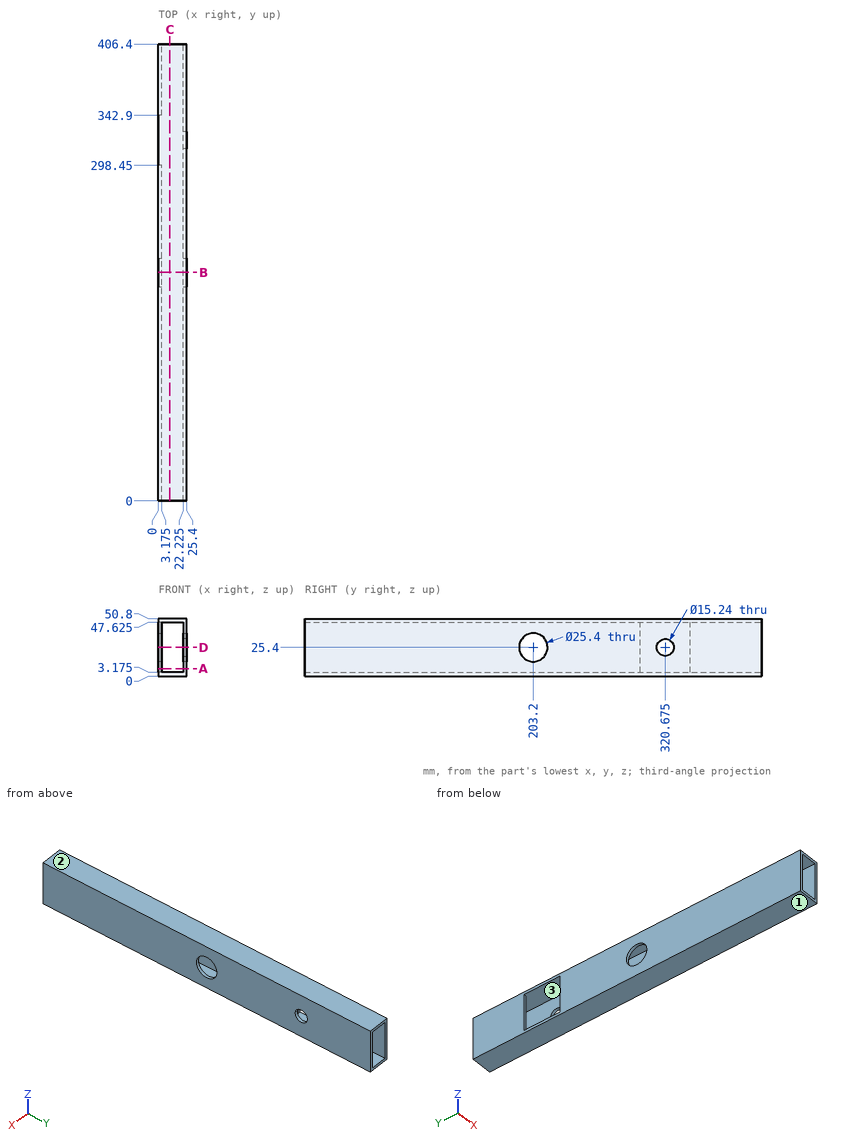
For this review, use the dimensioned drawing (mm, ordinates from the lowest corner) and the shaded views. Coordinates: 2 decimals unless noted, no trailing zeros. Loops run counter-clockwise (first coordinate to the right, second up) from the corner with the lowest first, then second, coordinate; pieces in that order, holes last. Notation, with made-up numbers: (1, -31.5) -> (57, -31.5) arc R21 ccw to (57, 7.5) -> close; hole circle Ø5 at (2, 30). An arc over 180 degrees is marked (long way). Use a Markdown table: item, result. Add a question column.
Item 1: The part is to be moulded in two halves that separate along Z. For the marked faces 1, 2 and 3, say which applies: +Z half, -Z half, draft (parallel to the pull), parting line (faces both ways), or undercut.
Item 2: We need section D-D, the plane z = 25.4. Write out the cut boundary in (x, y) (3 decimals), and give its area (3 significant figures).
Item 3: We need section C-C, the plane x = 10.25. Write out the cut boundary in (y, z) (3 decimals).
Item 4: Clearance check with a flat-ended pin moving along its axis: P1, Ø9, axis at y = 320.675, z = 25.4, coming from the -X side. State where the tip first meets the part, or that it passes through.
Item 5: We need section B-B, the plane y = 203.2. Write out the cut boundary in (x, z) (3 decimals).
Item 6: Wall thickness on L1, parallel to Y at x = 23.2, z = 25.4 (3 decimals); L2, parallel to Y at x = 1.2, z = 25.4; L3, parallel to Z at x = 5, y = 45.5 (3 decimals): over which ranges is each line inside the solid? List them lowest first. Write a range as from..to.
Item 7: We need section A-A, the plane z = 6.5. Write out the cut boundary in (x, y) (3 decimals), and give its area (3 significant figures).
Numbers:
| question | item | result |
|---|---|---|
| 1 | face 1 | -Z half |
| 1 | face 2 | +Z half |
| 1 | face 3 | undercut |
| 2 | outline | (0, 0) -> (3.175, 0) -> (3.175, 190.5) -> (0, 190.5) -> close; (0, 215.9) -> (3.175, 215.9) -> (3.175, 298.45) -> (0, 298.45) -> close; (0, 342.9) -> (3.175, 342.9) -> (3.175, 406.4) -> (0, 406.4) -> close; (22.225, 0) -> (25.4, 0) -> (25.4, 190.5) -> (22.225, 190.5) -> close; (22.225, 215.9) -> (25.4, 215.9) -> (25.4, 313.055) -> (22.225, 313.055) -> close; (22.225, 328.295) -> (25.4, 328.295) -> (25.4, 406.4) -> (22.225, 406.4) -> close |
| 2 | area | 2,230 mm^2 |
| 3 | outline | (0, 0) -> (406.4, 0) -> (406.4, 3.175) -> (0, 3.175) -> close; (0, 47.625) -> (406.4, 47.625) -> (406.4, 50.8) -> (0, 50.8) -> close |
| 4 | P1 | passes through |
| 5 | outline | (0, 0) -> (25.4, 0) -> (25.4, 12.7) -> (22.225, 12.7) -> (22.225, 3.175) -> (3.175, 3.175) -> (3.175, 12.7) -> (0, 12.7) -> close; (0, 38.1) -> (3.175, 38.1) -> (3.175, 47.625) -> (22.225, 47.625) -> (22.225, 38.1) -> (25.4, 38.1) -> (25.4, 50.8) -> (0, 50.8) -> close |
| 6 | L1 | y = 0..190.5, 215.9..313.055, 328.295..406.4 |
| 6 | L2 | y = 0..190.5, 215.9..298.45, 342.9..406.4 |
| 6 | L3 | z = 0..3.175, 47.625..50.8 |
| 7 | outline | (0, 0) -> (3.175, 0) -> (3.175, 298.45) -> (0, 298.45) -> close; (0, 342.9) -> (3.175, 342.9) -> (3.175, 406.4) -> (0, 406.4) -> close; (22.225, 0) -> (25.4, 0) -> (25.4, 406.4) -> (22.225, 406.4) -> close |
| 7 | area | 2,440 mm^2 |
